Geometry check sheet. Reference: the model listing, model coordinates, mm. A direction names the side the tool comes from. Coordinates: 2 decimals unless noted, no trailing zeros. Write each loop counter-clockwise with the first axis right and the second up, starting at its lowest first coordinate (ties: lowest second). Pieces come first, ordered by that corner, then holes. Notation, with made-up numbers: (15.5, 19) -> (29.5, 19) arc R28 cw to (29.5, 41) -> close; hole circle Ø1 at (85, 87.5). An arc over 180 degrees is marked (long way). Use a Markdown table: item, result.
Autodesk Inventor part; units mm, degrees
ref_plane "YZ Plane" through (0, 0, 0) normal (1, 0, 0) x (0, 1, 0)
ref_plane "XZ Plane" through (0, 0, 0) normal (0, 1, 0) x (-1, 0, 0)
ref_plane "XY Plane" through (0, 0, 0) normal (0, 0, 1) x (1, 0, 0)
sketch "Sketch1" plane through (0, 0, 0) normal (0, 0, 1) x (1, 0, 0)
  line L0 (0, 0) -> (0, 11.5)
  line L1 (0, 0) -> (-3.15, 0)
  line L2 (-3.15, 0) -> (-3.15, 1)
  arc A0 (-5, 3) -> (-3.15, 1) centre (-2.9939, 3) ccw
  line L3 (-5, 3) -> (-5, 8)
  arc A1 (-3, 10) -> (-5, 8) centre (-3, 8) ccw
  line L4 (-3, 10) -> (-2.3, 10)
  line L5 (-2.3, 10) -> (-2.3, 11.5)
  line L6 (-2.3, 11.5) -> (0, 11.5)
  dimension "d0" = 11.5
  dimension "d1" = 3.15
  dimension "d2" = 1
  dimension "d3" = 5
  dimension "d4" = 5
  dimension "d5" = 2.3
  dimension "d7" = 2
  dimension "d8" = 2
  dimension "d9" = 2
revolve "Revolution1" add sketch "Sketch1" angle 360 about axis through (0, 0, 0) along (0, 1, 0)
sketch "Sketch2" plane through (0, 0, 0) normal (0, -1, 0) x (1, 0, 0)
  circle A0 centre (0, 0) radius 2.5975
  dimension "d11" = 5.195
extrude "Extrusion1" cut sketch "Sketch2" against normal blind 8.6
sketch "Sketch3" plane through (0, 11.5, 0) normal (0, 1, 0) x (1, 0, 0)
  circle A0 centre (0, 0) radius 2.3
  circle A1 centre (0, 0) radius 1.6
  dimension "d14" = 0.7
extrude "Extrusion2" cut sketch "Sketch3" against normal blind 2.2 contours A1
sketch "Sketch4" plane through (0, 9.3, 0) normal (0, 1, 0) x (1, 0, 0)
  circle A0 centre (0, 0) radius 0.4 construction
  circle A1 centre (0, 0) radius 1.6
  line L0 (-1.5639, 0.338) -> (-0.2139, 0.338)
  line L1 (-0.2139, 0.338) -> (0.4734, 1.5284)
  arc A2 (0.4734, 1.5284) -> (-1.5639, 0.338) centre (0, 0) ccw
  dimension "d17" = 0.8
  dimension "d18" = 1.35
  dimension "d19" = 120
extrude "Extrusion3" cut sketch "Sketch4" against normal blind 4 contours L1 L0 A1 picked at (0.1203, 1.1544)
pattern_circular "Circular Pattern1" count 3 over 360 about axis through (0, 11.5, 0) along (0, -1, 0) of "Extrusion3"
sketch "Sketch5" plane through (0, 9.3, 0) normal (0, 1, 0) x (1, 0, 0)
  circle A0 centre (0, 0) radius 0.25
  dimension "d25" = 0.5
extrude "Extrusion4" cut sketch "Sketch5" against normal blind 0.2
properties part number "Lego head"
Item 1: Section check A-A on x = 0. Count the separate pieces of the cut face and the enclosed holes in it, then the cut area to 3 significant figures.
Answer block:
| item | result |
|---|---|
| separate pieces | 3 |
| enclosed holes | 0 |
| area | 46.7 mm^2 |
Item 2: Section check C-C on y = 3.5. Record the boundary of the cut face in (x, z) (1 decimal), then the cut area to 3 significant figures.
Answer block:
| item | result |
|---|---|
| outline | circle Ø10 at (0, 0); hole circle Ø5.2 at (0, 0) |
| area | 57.3 mm^2 |
Item 3: Section check B-B on y = 8.75. Record the boundary of the cut face in (x, z), then the cut area to 3 significant figures.
Answer block:
| item | result |
|---|---|
| outline | circle Ø9.71 at (0, 0); hole (-1.56, -0.34) arc R1.6 ccw to (0.47, -1.53) -> (-0.21, -0.34) -> close; hole (-1.56, 0.35) -> (-0.19, 0.35) -> (0.49, 1.52) arc R1.6 ccw to start; hole (0.4, -0.02) -> (1.07, -1.19) arc R1.6 ccw to (1.09, 1.17) -> close |
| area | 69.1 mm^2 |
Item 4: Depth check by flat-ended pin: P1, Ø0.8, axis at x = -1, y = 9, coming from the +Z side; P2, Ø1.6, axis at x = 0, z = 0.5, coming from the -Y side; P3, Ø2.5, axis at x = 0, z = 0, coming from the +Y side. Enter the tip coordinate at first touch or a pass-through.
Answer block:
| item | result |
|---|---|
| P1 | stops at z = 4.82 |
| P2 | stops at y = 8.6 |
| P3 | stops at y = 9.3 |
Item 5: Thickness scan on L1, parallel to Z at x = 0, y = 6.5; L2, parallel to Z at x = 0, y = 10.75; L3, parallel to X at y = 8.75, z = -0.5. Record the ranges inside material, lowest first. Write a range as [from, to].
Answer block:
| item | result |
|---|---|
| L1 | z = [-5, -2.6], [2.6, 5] |
| L2 | z = [-2.3, -1.6], [1.6, 2.3] |
| L3 | x = [-4.83, -1.52], [-0.12, 0.68], [1.52, 4.83] |
Item 6: Tool access check on faces 4 (the flat face through (-2, 10, -2)), 5 (the cylindrical face through (2.5, 0.507, -1.917)), 6 (the cylindrical face through (1.08, 5.54, -4.88)). Record the directions out of +Z, -Z, +X, -X, +Y, -Y that give a thin tool (end or side, any length) a straight path to the whole face; none if there is none.
Answer block:
| item | result |
|---|---|
| face 4 | +Y |
| face 5 | -Y |
| face 6 | +Y, -Y |
Item 7: Mould release check, pull along Z, two halves, no side actions. Record for faces 1 (the cylindrical face through (1.825, 10.76, -1.4)), 2 (the flat face through (0, 11.5, 2)), 3 (the cylindrical face through (-0.563, 4.24, -2.536)): +Z half, -Z half, draft (parallel to the pull), parting line (faces both ways), or undercut.
Answer block:
| item | result |
|---|---|
| face 1 | parting line |
| face 2 | draft |
| face 3 | undercut |
